```python
from build123d import *

# Parameters (mm, degrees)
SKETCH1_W                    = 210
SKETCH1_H                    = 75
SKETCH1_R                    = 11.9875
BASE_FLANGE1_DEPTH           = 3.175
EDGE_FLANGE1_STRIP_W         = 14.1732
EDGE_FLANGE1_STRIP_H         = 3.175
EDGE_FLANGE1_STRIP_CUT_DEPTH = 210
EDGE_FLANGE1_DEPTH           = 210
M6_CLEARANCE_HOLE2_D         = 6.4
M5_CLEARANCE_HOLE1_D         = 5.3
FILLET1_R                    = 5


# Sheet-metal steps are written as plain solids
with BuildPart() as part:
    # Sketch1 → Base-Flange1 (new body)
    with BuildSketch(Plane.XY):
        with Locations((35, 2.5)):
            Rectangle(SKETCH1_W, SKETCH1_H)
        Circle(SKETCH1_R, mode=Mode.SUBTRACT)
    extrude(amount=-BASE_FLANGE1_DEPTH)

    # Edge-Flange1 strip (across the edge) → Edge-Flange1 strip cut (cut)
    with BuildSketch(Plane(origin=(-70, 40, -3.175), x_dir=(0, -1, 0), z_dir=(1, 0, 0))):
        with Locations((-3.175, -1.5875)):
            Rectangle(EDGE_FLANGE1_STRIP_W, EDGE_FLANGE1_STRIP_H)
    extrude(amount=EDGE_FLANGE1_STRIP_CUT_DEPTH, mode=Mode.SUBTRACT)

    # Edge-Flange1 section (across the edge) → Edge-Flange1 (add)
    with BuildSketch(Plane(origin=(-70, 40, -3.175), x_dir=(0, -1, 0), z_dir=(1, 0, 0))):
        with BuildLine():
            Line((0, 0.7366), (0, 16.825))
            Line((0, 16.825), (3.175, 16.825))
            Line((3.175, 16.825), (3.175, 0.7366))
            ThreePointArc((3.175, 0.7366), (3.390745145, 0.215745145), (3.9116, 0))
            Line((3.9116, 0), (3.9116, -3.175))
            ThreePointArc((3.9116, -3.175), (1.145681115, -2.029318885), (0, 0.7366))
        make_face()
    extrude(amount=EDGE_FLANGE1_DEPTH)

    # M6 Clearance Hole2 (through all)
    with Locations(Plane(origin=(-50, 10, 0), x_dir=(1, 0, 0), z_dir=(0, 0, 1))):
        with Locations((0, 0), (0, -20), (170, -20), (170, 0)):
            Hole(M6_CLEARANCE_HOLE2_D / 2)

    # M5 Clearance Hole1 (through all)
    with Locations(Plane(origin=(-30, 25, 0), x_dir=(1, 0, 0), z_dir=(0, 0, 1))):
        with Locations((0, 0), (0, -50), (130, -50), (130, 0)):
            Hole(M5_CLEARANCE_HOLE1_D / 2)

    # Fillet1
    fillet1_edges = [part.edges().sort_by_distance(p)[0] for p in [
        (-70, 38.4125, -20),
        (140, 38.4125, -20),
        (140, -35, -1.5875),
        (-70, -35, -1.5875),
    ]]
    fillet(fillet1_edges, radius=FILLET1_R)


solid = part.part
```
Verification items for the finished model (mm, model axes). A direction names the side the tool comes from. Coordinates: 2 decimals unless noted, no trailing zeros. Write each loop counter-clockwise with the first axis right and the second up, starting at its lowest first coordinate (ties: lowest second). Pieces come first, ordered by that corner, then holes. Notation, with made-up numbers: (47, 57.5) - (97, 57.5) arc R24 cw to (97, 86.5) - close; hole circle Ø2 at (-12, -34.5). An arc over 180 degrees is marked (long way). Write item = value, one per line.
Q1. Cross-section at C-C (y = 0). Enter the section's corners in (x, z) (1 decimal), plus the area to 3 significant figures.
Answer:
outline = (-70, -3.2) - (-12, -3.2) - (-12, 0) - (-70, 0) - close; (12, -3.2) - (140, -3.2) - (140, 0) - (12, 0) - close
area = 591 mm²
Q2. Material ranges on L1, parallel to Z at x = 78.5, y = 11.5 (3 decimals); L2, parallel to Y at x = 26, z = -6.5 (3 decimals); L3, parallel to Y at x = 10.5, z = -1, recorded low to high. Write a range as from..to.
Answer:
L1 = -3.175..0
L2 = 36.825..40
L3 = -35..-5.78, 5.78..38.7
Q3. Cross-section at A-A (x = 0). Enter the section's corners in (y, z) (1 decimal).
Answer:
outline = (-35, -3.2) - (-12, -3.2) - (-12, 0) - (-35, 0) - close; (12, -3.2) - (36.1, -3.2) arc R0.7 cw to (36.8, -3.9) - (36.8, -20) - (40, -20) - (40, -3.9) arc R3.9 ccw to (36.1, 0) - (12, 0) - close
Q4. Cross-section at B-B (x = -50). Enter the section's corners in (y, z) (3 decimals), plus the area to 3 significant figures.
Answer:
outline = (-35, -3.175) - (-13.2, -3.175) - (-13.2, 0) - (-35, 0) - close; (-6.8, -3.175) - (6.8, -3.175) - (6.8, 0) - (-6.8, 0) - close; (13.2, -3.175) - (36.088, -3.175) arc R0.737 cw to (36.825, -3.912) - (36.825, -20) - (40, -20) - (40, -3.912) arc R3.912 ccw to (36.088, 0) - (13.2, 0) - close
area = 248 mm²
Q5. Access from +Z, -Z, +X, -X, +Y, -Y to the whole of each face (thin tool, end or side, straight path). Record for faces 1 (the face through (34, 1, -3.175)), 2 (the face through (98.777, -27.351, -1.61)).
Answer:
face_1 = -Z, +X, -X, -Y
face_2 = +Z, -Z
Q6. Mould release check, pull along X, two halves, no side actions. Record for faces 3 (the face through (34, 36.825, -12)), 4 (the face through (-8.835, 8.102, -1.565)), 5 (the face through (140, 7, -2)): released by +X, released by -X, zero draft, split by the parting line, or undercut.
Answer:
face_3 = zero draft
face_4 = undercut
face_5 = released by +X
Q7. Go/stop test with flat-tipped pins: pin 1 Ø2 at (y, z) = (-5, -5) entering from +X (3 decimals); pin 2 Ø2 at (x, y) = (8, -26) entering from +Z; pin 3 Ø5 at (x, z) = (13, -8.5) entering from -Y (3 decimals); pin 4 Ø8.5 at (x, y) = (100, 25) entering from -Z (3 decimals). Record where each tip stops, or that it passes through.
Answer:
pin_1 = through
pin_2 = 0
pin_3 = 36.825
pin_4 = -3.175
Q8. Cross-section at D-D (x = 112.5). Enter the section's corners in (y, z) (3 decimals), plus the area to 3 significant figures.
Answer:
outline = (-35, -3.175) - (36.088, -3.175) arc R0.737 cw to (36.825, -3.912) - (36.825, -20) - (40, -20) - (40, -3.912) arc R3.912 ccw to (36.088, 0) - (-35, 0) - close
area = 288 mm²
